Check sheet for the modelled part. Datum: model origin and axes. Units: mm. A direction names the side the tool comes from. Round coordinates to 2 decimals unless told otherwise and drop trailing zeros. Write each loop counter-clockwise with the first axis right and the second up, starting at its lowest first coordinate (ties: lowest second). Pieces come first, ordered by that corner, then holes.
Item 1: Depth check by flat-ended pin: pin 1 (1 mm diameter, centred on x = -6.5, z = 2, fed in from -Y); pin 2 (3 mm diameter, centred on y = 6.5, z = 2, fed in from -X); pin 3 (2 mm diameter, centred on x = -2, z = 1, fed in from -Y). Enter the tip coordinate at first touch or a pass-through.
Item 2: Section check A-A, the plane z = 7. Record the cut outline in (x, y).
Item 3: Section check B-B, the plane z = 1.25. Record the cut outline in (x, y), plus the area to 3 significant figures.
Item 4: Release check for a two-part mould opening along X. For faces 1 (the flat face through (-1, -11, 3.9)), 2 (the cylindrical face through (-1.264, 5.692, 6.986)), 3 (the cylindrical face through (-0.75, 3.4, 4.94)) record: pulls with the +X half, pulls with the -X half, needs draft (parallel to the pull), parting line crosses it, or undercut.
Item 5: Set-up check for faces 4 (the flat face through (4, -9, 3.65)), 5 (the flat face through (-3, 3, 0)): record each of +Z, -Z, +X, -X, +Y, -Y from which the full face is reachable in a straight line by a thin tool's end or side.
Item 6: Material ranges on line 1 along Y through (x, z) = (0, 6.75); line 2 along Z through (x, y) = (4.5, 4.5), recorded low to high.
from build123d import *

# Parameters (mm, degrees)
F2_SIZE  = 0.2
F3_R     = 1
F4_SIZE  = 0.5
F5_SIZE  = 0.5
F6_R     = 11.6305905431
F6_R_2   = 8.3305905431
F7_DEPTH = 0.25


# Not quite as in the source:
# - a fillet or chamfer that OpenCascade refuses, or shapes differently, is made with other operations: its cross-section is extruded or revolved along the edge and cut away or added


with BuildPart() as f1:
    # F0 (on Front) → F1 (revolve)
    with BuildSketch(Plane.XZ):
        Polygon((5.8305905431, 10), (3.48, 10), (3.48, 0), (5.8305905431, 0), (13.8305905431, 0), (13.3861808223, 1.95), (13.8305905431, 3.9), (5.8305905431, 3.9), align=None)
    revolve(axis=Axis((0, 0, 13.5622331873), (0, 0, -1)))

    # F2
    f2_edges = [f1.edges().sort_by_distance(p)[0] for p in [
        (-13.830591, 0, 3.9),
        (-13.830591, 0, 0),
    ]]
    chamfer(f2_edges, length=F2_SIZE)

    # F3
    f3_edges = [f1.edges().sort_by_distance(p)[0] for p in [
        (-13.386181, 0, 1.95),
    ]]
    fillet(f3_edges, radius=F3_R)

    # F4
    f4_edges = [f1.edges().sort_by_distance(p)[0] for p in [
        (-5.830591, 0, 10),
        (-3.48, 0, 10),
        (-5.830591, 0, 3.9),
    ]]
    chamfer(f4_edges, length=F4_SIZE)

    # F5
    f5_edges = [f1.edges().sort_by_distance(p)[0] for p in [
        (-3.48, 0, 0),
    ]]
    chamfer(f5_edges, length=F5_SIZE)

    # F6 (on face) → F7 (cut)
    with BuildSketch(Plane.XY.offset(3.9)):
        Circle(F6_R)
        Circle(F6_R_2, mode=Mode.SUBTRACT)
    extrude(amount=-F7_DEPTH, mode=Mode.SUBTRACT)

    # F8: chamfer of 1 on 2 edges, made by hand


with BuildPart() as f8_tool2:
    # F8_s3 → F8_t4 (revolve)
    with BuildSketch(Plane.XZ):
        Polygon((10.6305905431, 3.65), (11.6305905431, 4.65), (11.6305905431, 3.65), align=None)
    revolve(axis=Axis((0, 0, 3.65), (0, 0, 1)))

    split(bisect_by=Plane.XY.offset(3.9), keep=Keep.BOTTOM)


with BuildPart() as f1_1:
    add(f1.part)

    # F8_t1: union F8_tool2
    add(f8_tool2.part)


with BuildPart() as f8_tool7:
    # F8_s8 → F8_t9 (revolve)
    with BuildSketch(Plane.XZ):
        Polygon((8.3305905431, 4.65), (9.3305905431, 3.65), (8.3305905431, 3.65), align=None)
    revolve(axis=Axis((0, 0, 3.65), (0, 0, 1)))

    split(bisect_by=Plane.XY.offset(3.9), keep=Keep.BOTTOM)


with BuildPart() as f1_2:
    add(f1_1.part)

    # F8_t6: union F8_tool7
    add(f8_tool7.part)


solid = f1_2.part
Values found:
1. pin 1: stops at y = -12.01
1. pin 2: stops at x = -12.53
1. pin 3: stops at y = -13.71
2. outline: circle Ø11.66 at (0, 0); hole circle Ø6.96 at (0, 0)
3. outline: circle Ø27.09 at (0, 0); hole circle Ø6.96 at (0, 0)
3. area: 538 mm2
4. face 1: needs draft
4. face 2: parting line crosses it
4. face 3: undercut
5. face 4: +Z
5. face 5: -Z, +X, -X, +Y, -Y
6. line 1: y = -5.83 to -3.48, 3.48 to 5.83
6. line 2: z = 0 to 3.9
